Input: part model. Units: mm. Frame: model coordinates. A direction names the side the tool comes from. Give positions to 0.01 mm unless a question says otherwise; leave off trailing zeros. Loops run counter-clockwise (first coordinate to the right, second up) from the corner with the lowest first, then second, coordinate; pieces in that order, holes last. Notation, with made-up numbers: M -31.75,-18 L -2.75,-18 A28 cw -2.75,1 Z; hole C -26.75,-32 d8. An arc over 180 degrees is marked long. Use a Markdown table: item, result. Add a question column.
from build123d import *

# Parameters (mm, degrees)
F0_W     = 63.5
F0_H     = 63.5
F0_H_2   = 177.8
F0_R     = 31.75
F1_DEPTH = 184.15
F2_DEPTH = 120.65
F3_DEPTH = 63.5
F4_DEPTH = 38.1


with BuildPart() as f1:
    # F0 (on Top) → F1 (new body)
    with BuildSketch(Plane.XY):
        Polygon((-12.7, 152.4), (-127, 152.4), (-127, 50.8), (-44.45, 50.8), (-44.45, -50.8), (-127, -50.8), (-127, -152.4), (-12.7, -152.4), (-12.7, -88.9), (-12.7, 88.9), align=None)
        with Locations((19.05, 120.65)):
            Rectangle(F0_W, F0_H)
        with Locations((19.05, 0)):
            Rectangle(F0_W, F0_H_2)
        with Locations((19.05, -120.65)):
            Rectangle(F0_W, F0_H)
        with Locations((234.95, 0)):
            Rectangle(F0_W, F0_H_2)
        with Locations((234.95, 120.65)):
            Rectangle(F0_W, F0_H)
        with Locations((234.95, -120.65)):
            Rectangle(F0_W, F0_H)
        Polygon((381, 152.4), (266.7, 152.4), (266.7, 88.9), (266.7, -88.9), (266.7, -152.4), (381, -152.4), (381, -50.8), (298.45, -50.8), (298.45, 50.8), (381, 50.8), align=None)
        Polygon((203.2, 152.4), (50.8, 152.4), (50.8, 88.9), (50.8, -88.9), (50.8, -152.4), (203.2, -152.4), (203.2, -88.9), (203.2, 88.9), align=None)
        with Locations((127, 0)):
            Circle(F0_R, mode=Mode.SUBTRACT)
    extrude(amount=-F1_DEPTH)

    # F0 (on Top) → F2 (cut)
    with BuildSketch(Plane.XY):
        Polygon((-12.7, 152.4), (-127, 152.4), (-127, 50.8), (-44.45, 50.8), (-44.45, -50.8), (-127, -50.8), (-127, -152.4), (-12.7, -152.4), (-12.7, -88.9), (-12.7, 88.9), align=None)
        Polygon((381, 152.4), (266.7, 152.4), (266.7, 88.9), (266.7, -88.9), (266.7, -152.4), (381, -152.4), (381, -50.8), (298.45, -50.8), (298.45, 50.8), (381, 50.8), align=None)
    extrude(amount=-F2_DEPTH, mode=Mode.SUBTRACT)

    # F0 (on Top) → F3 (cut)
    with BuildSketch(Plane.XY):
        Polygon((203.2, 152.4), (50.8, 152.4), (50.8, 88.9), (50.8, -88.9), (50.8, -152.4), (203.2, -152.4), (203.2, -88.9), (203.2, 88.9), align=None)
        with Locations((127, 0)):
            Circle(F0_R, mode=Mode.SUBTRACT)
    extrude(amount=-F3_DEPTH, mode=Mode.SUBTRACT)

    # F0 (on Top) → F4 (cut)
    with BuildSketch(Plane.XY):
        with Locations((19.05, 0)):
            Rectangle(F0_W, F0_H_2)
        with Locations((234.95, 0)):
            Rectangle(F0_W, F0_H_2)
    extrude(amount=-F4_DEPTH, mode=Mode.SUBTRACT)


solid = f1.part
1) Contact query for flat-ended pins moving along their axis: P1, Ø6, axis at y = 43, z = -109, coming from the +X side; P2, Ø6, axis at y = 26, z = -85, coming from the -X side; P3, Ø5, axis at x = -20, y = -1, coming from the +Z side; P4, Ø19, axis at y = 11.5, z = -25, coming from the -X side. Output: stop coordinate, or through.
2) Reachability of faces 1 (the flat face through (19, 88.9, -19)), 2 (the flat face through (339, 50.8, -152)), 3 (the flat face through (-12.7, -2, -73)), 4 (the flat face through (-85, -50.8, -152)), 5 (the flat face through (203.2, -2.1, -38.4)) from +Z, -Z, +X, -X, +Y, -Y: full face, straight path, thin tool, end or side. Return the list, or none.
3) Section query D-D, the plane y = 0. Return the cut outline in (x, z), and give its area (3 significant figures).
4) Section query B-B, the plane x = 127. Return the cut outline in (y, z), and give its area (3 significant figures).
5) Ray query, line 1 (X direction, y = 131, z = -49); line 2 (Y direction, x = 127, z = -99); line 3 (Z direction, x = -86, y = 132.5). Return the intervals inside material, ascending. Write a range as [from, to].
6) Section query A-A, the plane z = -52. Return the cut outline in (x, y), and give its area (3 significant figures).
7) Pull-direction query (Y, two-part tool) for faces 6 (the flat face through (131, 152.4, -111)), 7 (the flat face through (19, 1, -38.1)), 8 (the flat face through (381, 101, -152)), 9 (the flat face through (-86, 50.8, -152)); classes: pulls with the +Y half, pulls with the -Y half, needs draft (parallel to the pull), parting line crosses it, or undercut.
8) Section query C-C, the plane z = -14. Return the cut outline in (x, y).
Entries:
| question | item | result |
|---|---|---|
| 1 | P1 | stops at x = 266.7 |
| 1 | P2 | stops at x = -12.7 |
| 1 | P3 | stops at z = -120.65 |
| 1 | P4 | passes through |
| 2 | face 1 | +Z, +X, -X |
| 2 | face 2 | +Z, -Z, +X |
| 2 | face 3 | +Z, -X, +Y, -Y |
| 2 | face 4 | +Z, -Z, -X |
| 2 | face 5 | +Z, +Y, -Y |
| 3 | outline | M -44.45,-184.15 L 95.25,-184.15 L 95.25,-63.5 L 50.8,-63.5 L 50.8,-38.1 L -12.7,-38.1 L -12.7,-120.65 L -44.45,-120.65 Z; M 158.75,-184.15 L 298.45,-184.15 L 298.45,-120.65 L 266.7,-120.65 L 266.7,-38.1 L 203.2,-38.1 L 203.2,-63.5 L 158.75,-63.5 Z |
| 3 | area | 33,300 mm² |
| 4 | outline | M -152.4,-184.15 L -31.75,-184.15 L -31.75,-63.5 L -152.4,-63.5 Z; M 31.75,-184.15 L 152.4,-184.15 L 152.4,-63.5 L 31.75,-63.5 Z |
| 4 | area | 29,100 mm² |
| 5 | line 1 | x = [-12.7, 50.8], [203.2, 266.7] |
| 5 | line 2 | y = [-152.4, -31.75], [31.75, 152.4] |
| 5 | line 3 | z = [-184.15, -120.65] |
| 6 | outline | M -12.7,-152.4 L 50.8,-152.4 L 50.8,152.4 L -12.7,152.4 Z; M 203.2,-152.4 L 266.7,-152.4 L 266.7,152.4 L 203.2,152.4 Z |
| 6 | area | 38,700 mm² |
| 7 | face 6 | pulls with the +Y half |
| 7 | face 7 | undercut |
| 7 | face 8 | needs draft |
| 7 | face 9 | undercut |
| 8 | outline | M -12.7,-152.4 L 50.8,-152.4 L 50.8,-88.9 L -12.7,-88.9 Z; M -12.7,88.9 L 50.8,88.9 L 50.8,152.4 L -12.7,152.4 Z; M 203.2,-152.4 L 266.7,-152.4 L 266.7,-88.9 L 203.2,-88.9 Z; M 203.2,88.9 L 266.7,88.9 L 266.7,152.4 L 203.2,152.4 Z |
